The listing builds one solid part. Answer for the finished solid, in the listing's coordinates (mm). Give positions to 0.01 mm unless a question says otherwise; leave off trailing zeros. Loops run counter-clockwise (first coordinate to the right, second up) from the corner with the lowest first, then second, coordinate; pieces in that order, holes last. Notation, with made-up numbers: (0, 4) - (58, 4) arc R22 ccw to (58, 29) - close; hole circle Ø3 at (-35.5, -26). An arc over 180 degrees is marked (long way). Write each question's results on one line, items separated by ' | '.
from build123d import *

# Parameters (mm, degrees)
SKETCH2_W           = 65
SKETCH2_H           = 25
SKETCH2_R           = 1
BOSS_EXTRUDE1_DEPTH = 2.3
FILLET9_R           = 10


with BuildPart() as part:
    # Sketch2 → Boss-Extrude1 (new body)
    with BuildSketch(Plane(origin=(0, 0, 0), x_dir=(1, 0, 0), z_dir=(0, 1, 0))):
        Rectangle(SKETCH2_W, SKETCH2_H)
        with Locations((0, -9.054487493)):
            Circle(SKETCH2_R, mode=Mode.SUBTRACT)
    extrude(amount=BOSS_EXTRUDE1_DEPTH)

    # Fillet9
    fillet9_edges = [part.edges().sort_by_distance(p)[0] for p in [
        (-32.5, 1.15, -12.5),
        (32.5, 1.15, -12.5),
    ]]
    fillet(fillet9_edges, radius=FILLET9_R)


solid = part.part
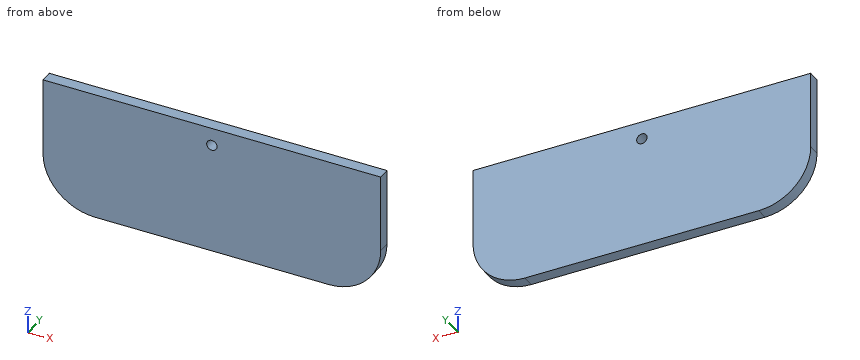
Item 1: Find the intervals of material crossed by line 1 along Z through (x, y) = (0, 1.4); line 2 along Z through (x, y) = (29.5, 1.35); line 3 along Z through (x, y) = (25.5, 0.5), in increasing order. Write a range as [from, to].
Values found:
line 1: z = [-12.5, 8.05], [10.05, 12.5] | line 2: z = [-9.64, 12.5] | line 3: z = [-12.04, 12.5]
Item 2: A cutting plane is placed at B-B, the plane y = 0.8. Determine the outline of the cut face in (x, z), plus the area to 3 significant figures.
Values found:
outline: (-32.5, -2.5) arc R10 ccw to (-22.5, -12.5) - (22.5, -12.5) arc R10 ccw to (32.5, -2.5) - (32.5, 12.5) - (-32.5, 12.5) - close; hole circle Ø2 at (0, 9.05) | area: 1,580 mm²
Item 3: A flat-ended cylindrical pin translates along its axis: P1, Ø8, axis at x = -10.5, z = -3, coming from the -Y side. Find the tip coordinate at first contact, or state that the pin passes through.
Values found:
P1: stops at y = 0
Item 4: A cutting plane is placed at A-A, the plane x = 0. Determine the outline of the cut face in (y, z).
Values found:
outline: (0, -12.5) - (2.3, -12.5) - (2.3, 8.05) - (0, 8.05) - close; (0, 10.05) - (2.3, 10.05) - (2.3, 12.5) - (0, 12.5) - close
